The model under review builds one solid part; all positions refer to its coordinate system, in mm. Coordinates: 2 decimals unless noted, no trailing zeros. Write each loop counter-clockwise with the first axis right and the second up, starting at its lowest first coordinate (ties: lowest second). Pieces come first, ordered by that corner, then holes.
1) For line 1 (X direction, y = -11, z = 30); line 2 (X direction, y = -10.5, z = 27.5); line 3 (Z direction, x = -204.5, y = -12.5), list the stretches that pass through material, from the lowest coordinate up.
2) For P1, Ø2, axis at x = -322.5, z = 23, coming from the +Y side; P2, Ø8, axis at x = -384.5, y = -5.5, coming from the -Z side, all flat-tipped, find the tip position at first contact; note any pin that passes through.
3) Add section C-C, the plane x = -360.5. State the section outline as (y, z) points, then the cut area to 3 significant figures.
4) Add section A-A, the plane x = -459. State the section outline as (y, z) points, then the cut area to 3 significant figures.
5) Add section D-D, the plane x = -320. State the section outline as (y, z) points, then the cut area to 3 significant figures.
6) Add section B-B, the plane z = 53. State the section outline as (x, y) points, then the cut area to 3 significant figures.
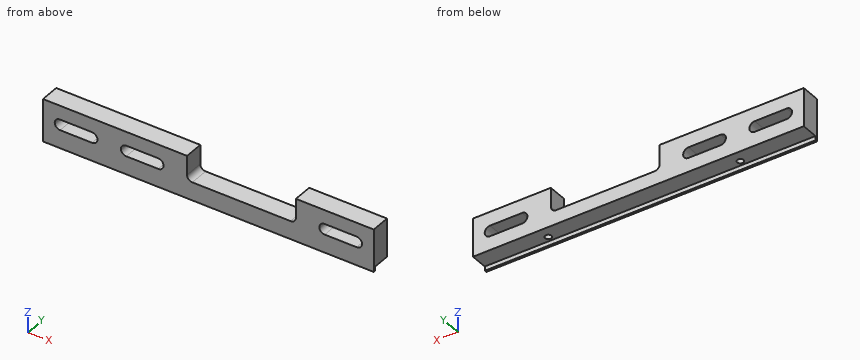
from build123d import *

# Parameters (mm, degrees)
F1_DEPTH = 18
F2_W     = 16
F2_H     = 4
F3_DEPTH = 400
F5_D     = 6
F5_DEPTH = 8
F5_TIP   = 1.8025818571


with BuildPart() as f1:
    # F0 (on Front) → F1 (new body)
    with BuildSketch(Plane.XZ):
        with BuildLine():
            Line((-489.9862787309, 20.9100212359), (-179.9862787309, 20.9100212359))
            Line((-179.9862787309, 20.9100212359), (-179.9862787309, 60.9100212359))
            Line((-179.9862787309, 60.9100212359), (-252.9862787309, 60.9100212359))
            Line((-252.9862787309, 60.9100212359), (-252.9862787309, 42.9100212359))
            ThreePointArc((-252.9862787309, 42.9100212359), (-254.450744825, 39.37448733), (-257.9862787309, 37.9100212359))
            Line((-257.9862787309, 37.9100212359), (-349.9862787309, 37.9100212359))
            ThreePointArc((-349.9862787309, 37.9100212359), (-353.5218126368, 39.37448733), (-354.9862787309, 42.9100212359))
            Line((-354.9862787309, 42.9100212359), (-354.9862787309, 60.9100212359))
            Line((-354.9862787309, 60.9100212359), (-489.9862787309, 60.9100212359))
            Line((-489.9862787309, 60.9100212359), (-489.9862787309, 20.9100212359))
        make_face()
        with BuildLine():
            Line((-443.9862787309, 37.9100212359), (-473.9862787309, 37.9100212359))
            ThreePointArc((-473.9862787309, 37.9100212359), (-478.9862787309, 42.9100212359), (-473.9862787309, 47.9100212359))
            Line((-473.9862787309, 47.9100212359), (-443.9862787309, 47.9100212359))
            ThreePointArc((-443.9862787309, 47.9100212359), (-438.9862787309, 42.9100212359), (-443.9862787309, 37.9100212359))
        make_face(mode=Mode.SUBTRACT)
        with BuildLine():
            Line((-381.9862787309, 37.9100212359), (-411.9862787309, 37.9100212359))
            ThreePointArc((-411.9862787309, 37.9100212359), (-416.9862787309, 42.9100212359), (-411.9862787309, 47.9100212359))
            Line((-411.9862787309, 47.9100212359), (-381.9862787309, 47.9100212359))
            ThreePointArc((-381.9862787309, 47.9100212359), (-376.9862787309, 42.9100212359), (-381.9862787309, 37.9100212359))
        make_face(mode=Mode.SUBTRACT)
        with BuildLine():
            Line((-195.9862787309, 37.9100212359), (-225.9862787309, 37.9100212359))
            ThreePointArc((-225.9862787309, 37.9100212359), (-230.9862787309, 42.9100212359), (-225.9862787309, 47.9100212359))
            Line((-225.9862787309, 47.9100212359), (-195.9862787309, 47.9100212359))
            ThreePointArc((-195.9862787309, 47.9100212359), (-190.9862787309, 42.9100212359), (-195.9862787309, 37.9100212359))
        make_face(mode=Mode.SUBTRACT)
    extrude(amount=F1_DEPTH)

    # F2 (on face) → F3 (cut)
    with BuildSketch(Plane.YZ.offset(-179.9862787309)):
        with Locations((-8, 22.9100212359)):
            Rectangle(F2_W, F2_H)
    extrude(amount=-F3_DEPTH, mode=Mode.SUBTRACT)

    # F5
    with Locations(Plane(origin=(0, 0, 24.9100212359), x_dir=(1, 0, 0), z_dir=(0, 0, -1))):
        with Locations((-242.9862787309, 11), (-422.9862787309, 11)):
            Hole(F5_D / 2, depth=F5_DEPTH)
            with Locations((0, 0, -(F5_DEPTH + F5_TIP / 2))):  # 118° drill point
                Cone(0, F5_D / 2, F5_TIP, mode=Mode.SUBTRACT)


solid = f1.part
Geometry results:
1. line 1: x = -489.99 to -425.99, -419.99 to -245.99, -239.99 to -179.99
1. line 2: x = -489.99 to -425.94, -420.03 to -245.94, -240.03 to -179.99
1. line 3: z = 24.91 to 37.91, 47.91 to 60.91
2. P1: stops at y = -16
2. P2: stops at z = 24.91
3. outline: (-18, 20.91) - (-16, 20.91) - (-16, 24.91) - (0, 24.91) - (0, 60.91) - (-18, 60.91) - close
3. area: 656 mm2
4. outline: (-18, 20.91) - (-16, 20.91) - (-16, 24.91) - (0, 24.91) - (0, 37.91) - (-18, 37.91) - close; (-18, 47.91) - (0, 47.91) - (0, 60.91) - (-18, 60.91) - close
4. area: 476 mm2
5. outline: (-18, 20.91) - (-16, 20.91) - (-16, 24.91) - (0, 24.91) - (0, 37.91) - (-18, 37.91) - close
5. area: 242 mm2
6. outline: (-489.99, -18) - (-354.99, -18) - (-354.99, 0) - (-489.99, 0) - close; (-252.99, -18) - (-179.99, -18) - (-179.99, 0) - (-252.99, 0) - close
6. area: 3,740 mm2
